Build history of the part. All positions in model axes, mm. A direction names the side the tool comes from. Round coordinates to 2 decimals unless told otherwise and drop trailing zeros. Write each loop counter-clockwise with the first axis right and the second up, starting at its lowest first coordinate (ties: lowest second). Pieces come first, ordered by that corner, then holes.
Item 1: Wall check: probe 1 along Y at (x, z) = (-4.85, 0); probe 2 along Z at (x, y) = (8.2, -3.9); probe 3 along Y at (x, z) = (9, 1.25). Give the ranges that are in metal, low to high.
Item 2: Band-saw the part on A-A, the plane x = 4.85. Write the cut outline in (y, z).
Item 3: Mould opens along X. For faces 1 (the flat face through (8.35, -3, 0)), 2 (the flat face through (1.05, -3, 0)), 3 (the flat face through (0, 3, -3.2)), 4 (the flat face through (-7.45, -3, 0)) say: +X half, -X half, draft (parallel to the pull), parting line (faces both ways), or undercut.
Item 4: Band-saw the part on C-C, the plane z = -2.5. Write the cut outline in (x, y), then the cut area to 3 significant figures.
Item 5: 3-axis set-ups, long thin cutter, end or side, ignore diameter. For faces 5 (the cylindrical face through (9.615, 6.199, -0.043)), 6 (the flat face through (9.9, 2, 0)), 7 (the flat face through (-9, 7, -3.1)), 8 (the flat face through (-2, 8, 1.9)): which of +Z, -Z, +X, -X, +Y, -Y reach the whole face in a straight line?
Item 6: Band-saw the part on B-B, the plane y = -3. Write the cut outline in (x, z), then the cut area to 3 significant figures.
Item 7: Drop flat-ended pins along their axis: pin 1 Ø8 at (x, y) = (11, -2.5) entering from -Z; pin 2 Ø1.4 at (y, z) = (-3.5, 0) entering from +X. Give the stop position or say it passes through.
Item 8: Band-saw the part on D-D, the plane z = 0. Count the separate pieces of the cut face and the enclosed holes in it, then the cut area to 3 significant figures.
```python
from build123d import *

# Parameters (mm, degrees)
SKETCH1_R                = 1.25
EXTRUDE1_DEPTH           = 3.2
EXTRUDE1_DEPTH_BACK      = 3.2
FILLET1_R                = 1
CUT_EXTRUDE1_DEPTH       = 0.1
CUT_EXTRUDE2_DEPTH       = 0.1
EXTRUDE3_DEPTH           = 1.75
EXTRUDE3_DEPTH_BACK      = 1.75
SKETCH6_R                = 0.6
CUT_EXTRUDE3_DEPTH       = 10.9
CUT_EXTRUDE3_DEPTH_BACK  = 10.9
SKETCH8_R                = 0.35
CUT_EXTRUDE4_DEPTH       = 0.1
SKETCH9_R                = 0.35
CUT_EXTRUDE5_DEPTH       = 0.1
EXTRUDE4_DEPTH           = 1.9
EXTRUDE4_DEPTH_BACK      = 1.9
EXTRUDE_THIN3_DEPTH      = 2.1
EXTRUDE_THIN3_DEPTH_BACK = 2.1
FILLET6_R                = 0.1
FILLET7_R                = 0.3


with BuildPart() as part:
    # Sketch1 → Extrude1 (new body, two sides)
    with BuildSketch(Plane.XY) as extrude1_sk:
        Polygon((-9.9, 7.5), (2.4, 7.5), (2.4, 6.5), (9.9, 6.5), (9.9, -2.5), (-9.9, -2.5), align=None)
        with Locations((-4.85, 0)):
            Circle(SKETCH1_R, mode=Mode.SUBTRACT)
        with Locations((4.85, 0)):
            Circle(SKETCH1_R, mode=Mode.SUBTRACT)
    extrude(amount=EXTRUDE1_DEPTH)
    extrude(extrude1_sk.sketch, amount=-EXTRUDE1_DEPTH_BACK)

    # Fillet1
    fillet1_edges = [part.edges().sort_by_distance(p)[0] for p in [
        (-9.9, 7.5, 0),
        (9.9, 6.5, 0),
    ]]
    fillet(fillet1_edges, radius=FILLET1_R)

    # Sketch2 → Cut-Extrude1 (cut)
    with BuildSketch(Plane.XY.offset(3.2)):
        with BuildLine():
            Line((8.9, 6.5), (4.024187691, 6.5))
            Line((4.024187691, 6.5), (4.024187691, 5.7))
            Line((4.024187691, 5.7), (8.9, 5.7))
            ThreePointArc((8.9, 5.7), (9.041421356, 5.641421356), (9.1, 5.5))
            Line((9.1, 5.5), (9.1, 4.482655552))
            Line((9.1, 4.482655552), (9.9, 4.482655552))
            Line((9.9, 4.482655552), (9.9, 5.5))
            ThreePointArc((9.9, 5.5), (9.607106781, 6.207106781), (8.9, 6.5))
        make_face()
        Polygon((9.9, -2.5), (9.9, 0), (9.1, 0), (9.1, -1.7), (9.1, -2.5), align=None)
        Polygon((-9.9, -2.5), (-9.1, -2.5), (-9.1, -1.7), (-9.1, 0), (-9.9, 0), align=None)
        with BuildLine():
            Line((-8.006418485, 7.5), (-8.9, 7.5))
            ThreePointArc((-8.9, 7.5), (-9.607106781, 7.207106781), (-9.9, 6.5))
            Line((-9.9, 6.5), (-9.9, 5.761874198))
            Line((-9.9, 5.761874198), (-9.1, 5.761874198))
            Line((-9.1, 5.761874198), (-9.1, 6.5))
            ThreePointArc((-9.1, 6.5), (-9.041421356, 6.641421356), (-8.9, 6.7))
            Line((-8.9, 6.7), (-8.006418485, 6.7))
            Line((-8.006418485, 6.7), (-8.006418485, 7.5))
        make_face()
    extrude(amount=-CUT_EXTRUDE1_DEPTH, mode=Mode.SUBTRACT)

    # Sketch3 → Cut-Extrude2 (cut)
    with BuildSketch(Plane(origin=(0, 0, -3.2), x_dir=(-1, 0, 0), z_dir=(0, 0, -1))):
        with BuildLine():
            Line((8.9, 7.5), (8.006418485, 7.5))
            Line((8.006418485, 7.5), (8.006418485, 6.7))
            Line((8.006418485, 6.7), (8.9, 6.7))
            ThreePointArc((8.9, 6.7), (9.041421356, 6.641421356), (9.1, 6.5))
            Line((9.1, 6.5), (9.1, 5.761874198))
            Line((9.1, 5.761874198), (9.9, 5.761874198))
            Line((9.9, 5.761874198), (9.9, 6.5))
            ThreePointArc((9.9, 6.5), (9.607106781, 7.207106781), (8.9, 7.5))
        make_face()
        Polygon((9.1, -1.7), (9.1, -2.5), (9.9, -2.5), (9.9, 0), (9.1, 0), align=None)
        Polygon((-9.9, 0), (-9.9, -2.5), (-9.1, -2.5), (-9.1, -1.7), (-9.1, 0), align=None)
        with BuildLine():
            Line((-4.024187691, 5.7), (-4.024187691, 6.5))
            Line((-4.024187691, 6.5), (-8.9, 6.5))
            ThreePointArc((-8.9, 6.5), (-9.607106781, 6.207106781), (-9.9, 5.5))
            Line((-9.9, 5.5), (-9.9, 4.482655552))
            Line((-9.9, 4.482655552), (-9.1, 4.482655552))
            Line((-9.1, 4.482655552), (-9.1, 5.5))
            ThreePointArc((-9.1, 5.5), (-9.041421356, 5.641421356), (-8.9, 5.7))
            Line((-8.9, 5.7), (-4.024187691, 5.7))
        make_face()
    extrude(amount=-CUT_EXTRUDE2_DEPTH, mode=Mode.SUBTRACT)

    # Sketch5 → Extrude3 (add, two sides)
    with BuildSketch(Plane.XY) as extrude3_sk:
        Polygon((-7.95, -2.5), (-7.7, -2.5), (-7.45, -2.5), (-7.45, -5.3), (-7.95, -5.3), align=None)
        Polygon((8.1, -2.5), (8.35, -2.5), (8.35, -5.3), (7.85, -5.3), (7.85, -2.5), align=None)
        Polygon((0.55, -2.5), (0.8, -2.5), (1.05, -2.5), (1.05, -5.3), (0.55, -5.3), align=None)
    extrude(amount=EXTRUDE3_DEPTH)
    extrude(extrude3_sk.sketch, amount=-EXTRUDE3_DEPTH_BACK)

    # Sketch6 → Cut-Extrude3 (cut, two sides)
    with BuildSketch(Plane(origin=(0, 0, 0), x_dir=(0, 0, -1), z_dir=(1, 0, 0))) as cut_extrude3_sk:
        with Locations((0, -3.9)):
            Circle(SKETCH6_R)
    extrude(amount=CUT_EXTRUDE3_DEPTH, mode=Mode.SUBTRACT)
    extrude(cut_extrude3_sk.sketch, amount=-CUT_EXTRUDE3_DEPTH_BACK, mode=Mode.SUBTRACT)

    # Sketch8 → Cut-Extrude4 (cut)
    with BuildSketch(Plane.XY.offset(3.2)):
        with Locations((-6.351950972, 6.27426345)):
            Circle(SKETCH8_R)
    extrude(amount=-CUT_EXTRUDE4_DEPTH, mode=Mode.SUBTRACT)

    # Sketch9 → Cut-Extrude5 (cut)
    with BuildSketch(Plane(origin=(0, 0, -3.2), x_dir=(-1, 0, 0), z_dir=(0, 0, -1))):
        with Locations((6.351950972, 6.27426345)):
            Circle(SKETCH9_R)
    extrude(amount=-CUT_EXTRUDE5_DEPTH, mode=Mode.SUBTRACT)

    # Sketch11 → Extrude4 (add, two sides)
    with BuildSketch(Plane.XY) as extrude4_sk:
        with BuildLine():
            Line((-2.73, 7.65), (-2.73, 6.9))
            Line((-2.73, 6.9), (-1.23, 6.9))
            Line((-1.23, 6.9), (-1.23, 7.65))
            ThreePointArc((-1.23, 7.65), (-1.98, 8.4), (-2.73, 7.65))
        make_face()
    extrude(amount=EXTRUDE4_DEPTH)
    extrude(extrude4_sk.sketch, amount=-EXTRUDE4_DEPTH_BACK)

    # Sketch12 → Extrude-Thin3 (add, two sides)
    with BuildSketch(Plane.XY) as extrude_thin3_sk:
        Polygon((-6.268968863, 7.489547154), (-6.173852185, 8.394521895), (18.1, 8.394521895), (18.1, 8.594521895), (-6.353932994, 8.594521895), (-6.467873242, 7.510452846), align=None)
    extrude(amount=EXTRUDE_THIN3_DEPTH)
    extrude(extrude_thin3_sk.sketch, amount=-EXTRUDE_THIN3_DEPTH_BACK)

    # Fillet6
    fillet6_edges = [part.edges().sort_by_distance(p)[0] for p in [
        (-6.173852185, 8.394521895, 0),
    ]]
    fillet(fillet6_edges, radius=FILLET6_R)

    # Fillet7
    fillet7_edges = [part.edges().sort_by_distance(p)[0] for p in [
        (-6.353932994, 8.594521895, 0),
    ]]
    fillet(fillet7_edges, radius=FILLET7_R)


solid = part.part
```
Results:
1. probe 1: y = -2.5 to -1.25, 1.25 to 7.5, 8.39 to 8.59
1. probe 2: z = -1.75 to -0.6, 0.6 to 1.75
1. probe 3: y = -2.5 to 6.49, 8.39 to 8.59
2. outline: (-2.5, -3.2) - (-1.25, -3.2) - (-1.25, 3.2) - (-2.5, 3.2) - close; (1.25, -3.2) - (5.7, -3.2) - (5.7, -3.1) - (6.5, -3.1) - (6.5, 3.1) - (5.7, 3.1) - (5.7, 3.2) - (1.25, 3.2) - close; (8.39, -2.1) - (8.59, -2.1) - (8.59, 2.1) - (8.39, 2.1) - close
3. face 1: +X half
3. face 2: undercut
3. face 3: draft
3. face 4: undercut
4. outline: (-9.9, -2.5) - (9.9, -2.5) - (9.9, 5.5) arc R1 ccw to (8.9, 6.5) - (2.4, 6.5) - (2.4, 7.5) - (-8.9, 7.5) arc R1 ccw to (-9.9, 6.5) - close; hole circle Ø2.5 at (-4.85, 0); hole circle Ø2.5 at (4.85, 0)
4. area: 180 mm2
5. face 5: +Z, -Z, +X
5. face 6: +Z, -Z, +X, -Y
5. face 7: -Z, -X, +Y
5. face 8: +Z, +X
6. outline: (-7.95, -1.75) - (-7.45, -1.75) - (-7.45, 1.75) - (-7.95, 1.75) - close; (0.55, -1.75) - (1.05, -1.75) - (1.05, 1.75) - (0.55, 1.75) - close; (7.85, -1.75) - (8.35, -1.75) - (8.35, 1.75) - (7.85, 1.75) - close
6. area: 5.25 mm2
7. pin 1: stops at z = -3.2
7. pin 2: stops at x = 8.35
8. separate pieces: 4
8. enclosed holes: 3
8. area: 189 mm2
